Geometry: final body of the model. Coordinates: model frame, mm. A direction names the side the tool comes from. Round coordinates to 2 decimals unless told otherwise and drop trailing zeros. Put each result on its own line as item: value. Start each with the question number.
(1) Pin query (flat end, axial travel): P1, Ø8, axis at y = -33, z = 8.5, coming from the -X side; P2, Ø5, axis at y = 4.5, z = 7, coming from the +X side; P3, Ø10.5, axis at x = -300, y = 28, coming from the +Z side; P4, Ø1.5, axis at x = 187, y = 25, coming from the -Z side. Return the tip coordinate at first contact, or that it passes through.
(2) Access query for faces 1 (the face through (56, 1, 15)), 2 (the face through (1129.02, 0.92, 10.32)). Directions: +Z, -Z, +X, -X, +Y, -Y. A direction counts if a zero-diameter tool reaches every point of the face in a straight line with its end or side. Return the directions, or none.
(3) Section A-A (z = 7.75). Count the separate pieces of the cut face and the enclosed holes in it, and give its area (3 significant figures).
(4) Pull-direction query (X, two-part tool) for faces 3 (the face through (1189.99, 0.88, 7.4)), 4 (the face through (56, 1, 0)), 5 (the face through (1164, -9, 5.5)); classes: released by +X, released by -X, zero draft, split by the parting line, or undercut.
(5) Material intervals for L1, parallel to Y at x = 600, z = 7.5; L2, parallel to X at y = -11, z = 8.75; L3, parallel to X at y = 4.5, z = 10, sorted ascending. Write a range as [from, to].
from build123d import *

# Parameters (mm, degrees)
ESTRUSIONE1_DEPTH                    = 15
SCHIZZO2_R                           = 4
SCHIZZO2_R_2                         = 15
TAGLIO_ESTRUSIONE1_DEPTH             = 15
SCHIZZO4_R                           = 6.75
TAGLIO_ESTRUSIONE3_DEPTH             = 8.5
SCHIZZO5_R                           = 4
TAGLIO_ESTRUSIONE4_DEPTH             = 30
SMUSSO1_SIZE                         = 3
TAGLIO_ESTRUSIONE8_START             = -30
TAGLIO_ESTRUSIONE8_DEPTH             = 30
SCHIZZO12_R                          = 4
TAGLIO_ESTRUSIONE9_DEPTH             = 30
SCHIZZO13_R                          = 21
TAGLIO_ESTRUSIONE10_DEPTH            = 9.5
RIPETIZIONE_A_L1_COUNT               = 4
RIPETIZIONE_A_L1_PITCH               = 300
SMUSSO1_OF_RIPETIZIONE_A_L1_SIZE     = 3
RIPETIZIONE_A_L1_COL_COUNT           = 4
RIPETIZIONE_A_L1_COL_PITCH           = 300
SMUSSO1_OF_RIPETIZIONE_A_L1_COL_SIZE = 3
FORO_FILETTATO_M6_1_D                = 5


with BuildPart() as part:
    # Schizzo1 → Estrusione1 (new body)
    with BuildSketch(Plane.XY):
        with BuildLine():
            Line((-1150, 40), (1150, 40))
            ThreePointArc((1150, 40), (1190, 0), (1150, -40))
            Line((1150, -40), (-1150, -40))
            ThreePointArc((-1150, -40), (-1190, 0), (-1150, 40))
        make_face()
    extrude(amount=ESTRUSIONE1_DEPTH)

    # Schizzo2 → Taglio-Estrusione1 (cut)
    with BuildSketch(Plane.XY.offset(15)):
        with Locations((-1150, 0)):
            Circle(SCHIZZO2_R)
        with Locations(Location((1150, 0, 0), (0, 0, 180))):
            Circle(SCHIZZO2_R_2)
    extrude(amount=-TAGLIO_ESTRUSIONE1_DEPTH, mode=Mode.SUBTRACT)

    # Schizzo4 → Taglio-Estrusione3 (cut)
    with BuildSketch(Plane.XY.offset(15)):
        with Locations((-1150, 0)):
            Circle(SCHIZZO4_R)
    extrude(amount=-TAGLIO_ESTRUSIONE3_DEPTH, mode=Mode.SUBTRACT)

    # Schizzo5 → Taglio-Estrusione4 (cut)
    with BuildSketch(Plane.XY.offset(15)):
        with Locations((0, -2)):
            Circle(SCHIZZO5_R)
        with Locations((0, 28)):
            Circle(SCHIZZO5_R)
    taglio_estrusione4 = extrude(amount=-TAGLIO_ESTRUSIONE4_DEPTH, mode=Mode.SUBTRACT)

    # Smusso1
    smusso1_edges = [part.edges().sort_by_distance(p)[0] for p in [
        (-4, -2, 15),
        (-4, 28, 15),
    ]]
    chamfer(smusso1_edges, length=SMUSSO1_SIZE)

    # Schizzo11 → Taglio-Estrusione8 (cut)
    with BuildSketch(Plane.XY.offset(15).offset(TAGLIO_ESTRUSIONE8_START)):
        with BuildLine():
            Line((-1150, 40), (-1111, 40))
            Line((-1111, 40), (-1111, -20))
            ThreePointArc((-1111, -20), (-1109.535533906, -23.535533906), (-1106, -25))
            Line((-1106, -25), (-1016, -25))
            ThreePointArc((-1016, -25), (-1012.464466094, -26.464466094), (-1011, -30))
            Line((-1011, -30), (-1011, -40))
            Line((-1011, -40), (-1150, -40))
            ThreePointArc((-1150, -40), (-1190, 0), (-1150, 40))
        make_face()
    extrude(amount=TAGLIO_ESTRUSIONE8_DEPTH, mode=Mode.SUBTRACT)

    # Schizzo12 → Taglio-Estrusione9 (cut)
    with BuildSketch(Plane.XZ.offset(25)):
        with Locations(Location((-1095, 7.5, 0), (0, 0, 270))):
            Circle(SCHIZZO12_R)
        with Locations(Location((-1045, 7.5, 0), (0, 0, 270))):
            Circle(SCHIZZO12_R)
    extrude(amount=-TAGLIO_ESTRUSIONE9_DEPTH, mode=Mode.SUBTRACT)

    # Schizzo13 → Taglio-Estrusione10 (cut)
    with BuildSketch(Plane.XY.offset(15)):
        with Locations((1150, 0)):
            Circle(SCHIZZO13_R)
    extrude(amount=-TAGLIO_ESTRUSIONE10_DEPTH, mode=Mode.SUBTRACT)

    # Ripetizione a L1: Taglio-Estrusione4 ×4
    with Locations(*[(-i * RIPETIZIONE_A_L1_PITCH, 0, 0) for i in range(1, RIPETIZIONE_A_L1_COUNT)]):
        add(taglio_estrusione4, mode=Mode.SUBTRACT)

    # Smusso1 of Ripetizione a L1
    smusso1_of_ripetizione_a_l1_edges = [part.edges().sort_by_distance(p)[0] for p in [
        (-304, -2, 15),
        (-304, 28, 15),
        (-604, -2, 15),
        (-604, 28, 15),
        (-904, -2, 15),
        (-904, 28, 15),
    ]]
    chamfer(smusso1_of_ripetizione_a_l1_edges, length=SMUSSO1_OF_RIPETIZIONE_A_L1_SIZE)

    # Ripetizione a L1 col: Taglio-Estrusione4 ×4
    with Locations(*[(i * RIPETIZIONE_A_L1_COL_PITCH, 0, 0) for i in range(1, RIPETIZIONE_A_L1_COL_COUNT)]):
        add(taglio_estrusione4, mode=Mode.SUBTRACT)

    # Smusso1 of Ripetizione a L1 col
    smusso1_of_ripetizione_a_l1_col_edges = [part.edges().sort_by_distance(p)[0] for p in [
        (296, -2, 15),
        (296, 28, 15),
        (596, -2, 15),
        (596, 28, 15),
        (896, -2, 15),
        (896, 28, 15),
    ]]
    chamfer(smusso1_of_ripetizione_a_l1_col_edges, length=SMUSSO1_OF_RIPETIZIONE_A_L1_COL_SIZE)

    # Foro filettato M6-1 (through all)
    with Locations(Plane.XY.offset(15)):
        with Locations((1127.019029611, 22.980970389), (1172.980970389, -22.980970389)):
            Hole(FORO_FILETTATO_M6_1_D / 2)


solid = part.part
Checks:
1. P1: stops at x = -1011.1
1. P2: stops at x = 1189.95
1. P3: stops at z = 13.25
1. P4: stops at z = 0
2. face 1: +Z, +X, -X, +Y, -Y
2. face 2: +Z
3. separate pieces: 1
3. enclosed holes: 17
3. area: 179,000 mm²
4. face 3: released by +X
4. face 4: zero draft
4. face 5: undercut
5. L1: y = [-40, -6], [2, 24], [32, 40]
5. L2: x = [-1111, -1098.8], [-1091.2, -1048.8], [-1041.2, 1132.11], [1167.89, 1188.46]
5. L3: x = [-1111, -1098.12], [-1091.88, -1048.12], [-1041.88, 1129.49], [1170.51, 1189.75]
